from build123d import *

# Parameters (mm, degrees)
SKETCH2_R           = 11.1125
BOSS_EXTRUDE1_DEPTH = 31.75
SKETCH3_R           = 6.35
CUT_EXTRUDE1_DEPTH  = 32.75
SKETCH4_W           = 3.175
SKETCH4_H           = 0.79375
CHAMFER1_SIZE       = 0.396875
SKETCH5_W           = 3.175
SKETCH5_H           = 1.190625


with BuildPart() as part:
    # Sketch2 → Boss-Extrude1 (new body)
    with BuildSketch(Plane.XY):
        Circle(SKETCH2_R)
    extrude(amount=BOSS_EXTRUDE1_DEPTH)

    # Sketch3 → Cut-Extrude1 (cut, through all)
    with BuildSketch(Plane.XY.offset(31.75)):
        Circle(SKETCH3_R)
    extrude(amount=-CUT_EXTRUDE1_DEPTH, mode=Mode.SUBTRACT)

    # Sketch4 → Cut-Revolve1 (revolve, cut)
    with BuildSketch(Plane(origin=(0, 0, 0), x_dir=(1, 0, 0), z_dir=(0, 1, 0))):
        with Locations((11.1125, -26.9875)):
            Rectangle(SKETCH4_W, SKETCH4_H)
        with Locations((11.1125, -4.7625)):
            Rectangle(SKETCH4_W, SKETCH4_H)
    revolve(axis=Axis((0, 0, 31.75), (0, 0, -1)), mode=Mode.SUBTRACT)

    # Chamfer1
    chamfer1_edges = [part.edges().sort_by_distance(p)[0] for p in [
        (-11.1125, 0, 0),
        (-11.1125, 0, 31.75),
    ]]
    chamfer(chamfer1_edges, length=CHAMFER1_SIZE)

    # Sketch5 → Cut-Revolve2 (revolve, cut)
    with BuildSketch(Plane(origin=(0, 0, 0), x_dir=(1, 0, 0), z_dir=(0, 1, 0))):
        with Locations((11.1125, -12.7)):
            Rectangle(SKETCH5_W, SKETCH5_H)
        with Locations((11.1125, -19.137777624)):
            Rectangle(SKETCH5_W, SKETCH5_H)
    revolve(axis=Axis((0, 0, 31.75), (0, 0, -1)), mode=Mode.SUBTRACT)


solid = part.part
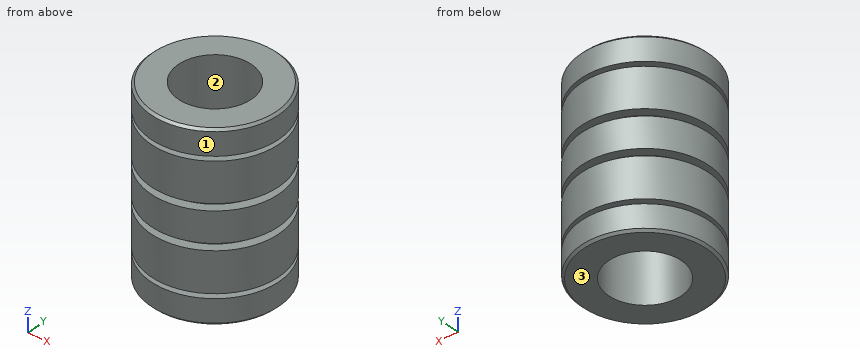
Geometry: final body of the model. Coordinates: model frame, mm. Face numbers are marked on the shaded views. Give positions to 0.01 mm unless a question says otherwise; leave off trailing zeros. Loops run counter-clockwise (first coordinate to the right, second up) from the corner with the lowest first, then second, coordinate; pieces in that order, holes last. Notation, with made-up numbers: M -15,66.5 L 29,66.5 A12 ccw 29,76.5 Z; hole C 33,89 d8. An arc over 180 degrees is marked long. Put each result on its own line as item: value. Start each with the question number.
1) Cut plane A-A (z = 12.5). Output: boundary loops of the cut face in (x, y) (3 decimals).
2) Contact query for flat-ended pins moving along their axis: pin 1 (2 mm diameter, centred on y = -6.5, z = 13, fed in from +X); pin 2 (1 mm diameter, centred on x = 5, z = 16.5, fed in from -Y); pin 3 (6 mm diameter, centred on x = -8, z = 4, fed in from -Y). Output: stop coordinate, or through.
3) Ray query, line 1 along Z through (x, y) = (-4.75, -9.5); line 2 along Y through (x, z) = (0, 16.5); line 3 along Y through (x, z) = (-4.75, 15). Return the intervals inside material, ascending.
4) Pull-direction query (X, two-part tool) for the marked faces 1, 2 and 3; classes: pulls with the +X half, pulls with the -X half, needs draft (parallel to the pull), parting line crosses it, or undercut.
Verdict:
1. outline: C 0,0 d19.05; hole C 0,0 d12.7
2. pin 1: x = 9.63
2. pin 2: y = -10.16
2. pin 3: y = -9.92
3. line 1: 0 to 4.37, 5.16 to 12.1, 13.3 to 18.54, 19.73 to 26.59, 27.38 to 31.75
3. line 2: -11.11 to -6.35, 6.35 to 11.11
3. line 3: -10.05 to -4.21, 4.21 to 10.05
4. face 1: parting line crosses it
4. face 2: undercut
4. face 3: needs draft
